Design review of the part built by this model. Coordinates are the model's own, in mm. Face numbers are marked on the shaded views. A direction names the side the tool comes from. Coordinates: 2 decimals unless noted, no trailing zeros. Write each loop counter-clockwise with the first axis right and the second up, starting at its lowest first coordinate (ties: lowest second). Pieces come first, ordered by that corner, then holes.
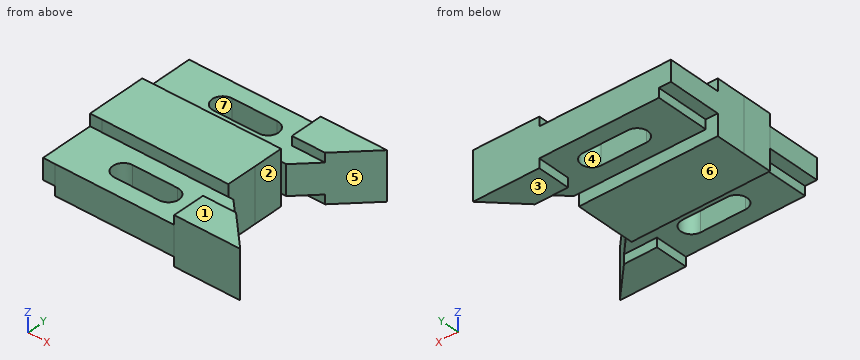
```python
from build123d import *

# Parameters (mm, degrees)
F0_W     = 6.35
F0_H     = 28.575
F1_DEPTH = 28.448
F3_DEPTH = 1.524
F4_DEPTH = 1.524
F5_DEPTH = 6.35
F6_DEPTH = 11.176
F7_DEPTH = 11.176
F2_W     = 6.35
F2_H     = 28.575
F8_DEPTH = 6.35


with BuildPart() as f1:
    # F0 (on Top) → F1 (new body)
    with BuildSketch(Plane.XY):
        Polygon((6.53696, 60.324607), (0.18696, 60.324607), (0.18696, 44.449607), (0.120189, 28.574747), (6.470133, 28.548039), (73.525377, 28.265996), (73.592798, 44.295231), (73.592798, 60.324607), align=None)
        Polygon((69.78296, 88.899607), (6.53696, 88.899607), (6.53696, 60.324607), (73.592798, 60.324607), (76.25996, 60.324607), (87.30896, 71.373607), (69.78296, 71.373607), align=None)
        with BuildLine():
            ThreePointArc((30.41296, 69.024107), (24.82496, 74.612107), (30.41296, 80.200107))
            Line((30.41296, 80.200107), (54.28896, 80.200107))
            ThreePointArc((54.28896, 80.200107), (59.87696, 74.612107), (54.28896, 69.024107))
            Line((54.28896, 69.024107), (30.41296, 69.024107))
        make_face(mode=Mode.SUBTRACT)
        with Locations((3.36196, 74.612107)):
            Rectangle(F0_W, F0_H)
        Polygon((73.525377, 28.265996), (6.470133, 28.548039), (6.349944, -0.026709), (69.595384, -0.292727), (69.6691, 17.233118), (87.194945, 17.159402), (76.192516, 28.254778), align=None)
        with BuildLine():
            Line((54.138112, 8.471865), (30.262323, 8.57229))
            ThreePointArc((30.262323, 8.57229), (24.697876, 14.183744), (30.309331, 19.748191))
            Line((30.309331, 19.748191), (54.185119, 19.647767))
            ThreePointArc((54.185119, 19.647767), (59.749566, 14.036312), (54.138112, 8.471865))
        make_face(mode=Mode.SUBTRACT)
        Polygon((69.6691, 17.233118), (69.595384, -0.292727), (104.647074, -0.440158), (87.194945, 17.159402), align=None)
        Polygon((6.470133, 28.548039), (0.120189, 28.574747), (0, 0), (6.349944, -0.026709), align=None)
        Polygon((104.83496, 88.899607), (69.78296, 88.899607), (69.78296, 71.373607), (87.30896, 71.373607), align=None)
    extrude(amount=F1_DEPTH)

    # F2 (on face) → F3 (cut)
    with BuildSketch(Plane.XY.offset(28.448)):
        Polygon((104.647074, -0.440158), (87.194945, 17.159402), (69.6691, 17.233118), (69.595384, -0.292727), align=None)
        Polygon((69.78296, 71.373607), (87.30896, 71.373607), (104.83496, 88.899607), (69.78296, 88.899607), align=None)
    extrude(amount=-F3_DEPTH, mode=Mode.SUBTRACT)

    # F0 (on Top) → F4 (cut)
    with BuildSketch(Plane.XY):
        Polygon((69.6691, 17.233118), (69.595384, -0.292727), (104.647074, -0.440158), (87.194945, 17.159402), align=None)
        Polygon((104.83496, 88.899607), (69.78296, 88.899607), (69.78296, 71.373607), (87.30896, 71.373607), align=None)
    extrude(amount=F4_DEPTH, mode=Mode.SUBTRACT)

    # F0 (on Top) → F5 (cut)
    with BuildSketch(Plane.XY):
        Polygon((73.525377, 28.265996), (6.470133, 28.548039), (6.349944, -0.026709), (69.595384, -0.292727), (69.6691, 17.233118), (87.194945, 17.159402), (76.192516, 28.254778), align=None)
        with BuildLine():
            Line((54.138112, 8.471865), (30.262323, 8.57229))
            ThreePointArc((30.262323, 8.57229), (24.697876, 14.183744), (30.309331, 19.748191))
            Line((30.309331, 19.748191), (54.185119, 19.647767))
            ThreePointArc((54.185119, 19.647767), (59.749566, 14.036312), (54.138112, 8.471865))
        make_face(mode=Mode.SUBTRACT)
        Polygon((69.78296, 88.899607), (6.53696, 88.899607), (6.53696, 60.324607), (73.592798, 60.324607), (76.25996, 60.324607), (87.30896, 71.373607), (69.78296, 71.373607), align=None)
        with BuildLine():
            ThreePointArc((30.41296, 69.024107), (24.82496, 74.612107), (30.41296, 80.200107))
            Line((30.41296, 80.200107), (54.28896, 80.200107))
            ThreePointArc((54.28896, 80.200107), (59.87696, 74.612107), (54.28896, 69.024107))
            Line((54.28896, 69.024107), (30.41296, 69.024107))
        make_face(mode=Mode.SUBTRACT)
        Polygon((6.470133, 28.548039), (0.120189, 28.574747), (0, 0), (6.349944, -0.026709), align=None)
        with Locations((3.36196, 74.612107)):
            Rectangle(F0_W, F0_H)
    extrude(amount=F5_DEPTH, mode=Mode.SUBTRACT)

    # F0 (on Top) → F6 (join)
    with BuildSketch(Plane.XY):
        Polygon((6.470133, 28.548039), (0.120189, 28.574747), (0, 0), (6.349944, -0.026709), align=None)
        with Locations((3.36196, 74.612107)):
            Rectangle(F0_W, F0_H)
    extrude(amount=F6_DEPTH)

    # F0 (on Top) → F7 (cut)
    with BuildSketch(Plane.XY):
        Polygon((6.470133, 28.548039), (0.120189, 28.574747), (0, 0), (6.349944, -0.026709), align=None)
        with Locations((3.36196, 74.612107)):
            Rectangle(F0_W, F0_H)
    extrude(amount=F7_DEPTH, mode=Mode.SUBTRACT)

    # F2 (on face) → F8 (cut)
    with BuildSketch(Plane.XY.offset(28.448)):
        Polygon((69.6691, 17.233118), (87.194945, 17.159402), (76.192516, 28.254778), (73.525377, 28.265996), (6.470133, 28.548039), (6.349944, -0.026709), (69.595384, -0.292727), align=None)
        with BuildLine():
            Line((30.309331, 19.748191), (54.185119, 19.647767))
            ThreePointArc((54.185119, 19.647767), (59.749566, 14.036312), (54.138112, 8.471865))
            Line((54.138112, 8.471865), (30.262323, 8.57229))
            ThreePointArc((30.262323, 8.57229), (24.697876, 14.183744), (30.309331, 19.748191))
        make_face(mode=Mode.SUBTRACT)
        Polygon((6.53696, 60.324607), (73.592798, 60.324607), (76.25996, 60.324607), (87.30896, 71.373607), (69.78296, 71.373607), (69.78296, 88.899607), (6.53696, 88.899607), align=None)
        with BuildLine():
            ThreePointArc((30.41296, 69.024107), (24.82496, 74.612107), (30.41296, 80.200107))
            Line((30.41296, 80.200107), (54.28896, 80.200107))
            ThreePointArc((54.28896, 80.200107), (59.87696, 74.612107), (54.28896, 69.024107))
            Line((54.28896, 69.024107), (30.41296, 69.024107))
        make_face(mode=Mode.SUBTRACT)
        Polygon((0, 0), (6.349944, -0.026709), (6.470133, 28.548039), (0.120189, 28.574747), align=None)
        with Locations((3.36196, 74.612107)):
            Rectangle(F2_W, F2_H)
    extrude(amount=-F8_DEPTH, mode=Mode.SUBTRACT)


solid = f1.part
```
(1) Consider section A-A (z = 3.5). Give the boundary of the cut face in (x, y).
(2) Consider section C-C (z = 14). Give the boundary of the cut face in (x, y).
(3) Wall thickness on line 1 (Y direction, x = 74.5, z = 11.75); line 2 (Y direction, x = 49, z = 17.5); line 3 (Z direction, x = 96.5, y = 85.5): over which ranges is each line inside the solid? List them lowest first.
(4) Mouldability with a two-part tool opening along X and no side actions: class the marked faces 5, 6 and 7 as +X half, -X half, draft (parallel to the pull), parting line (faces both ways), or undercut.
(5) Insertion check: pin 1 Ø3 at (y, z) = (65.5, 19.5) entering from -X; pin 2 Ø2.5 at (y, z) = (78.5, 4.5) entering from -X; pin 3 Ø10 at (x, y) = (81.5, 55) entering from -Z; pin 4 Ø9 at (x, y) = (81, 76.5) entering from +Z. Each pin has a flat end and moves straight along its axis. Give the tip position at first contact, or say it passes through.
(6) Consider section D-D (y = 74.5). Give the boundary of the cut face in (x, z), plus the area to 3 significant figures.
(7) Consider section B-B (x = 37). Give the boundary of the cut face in (y, z), plus the area to 3 significant figures.
(8) For the marked faces 1, 2, 3 and 4, list the 3-axis set-ups (+Z, -Z, +X, -X, +Y, -Y) from which the entire face can be reached by the end or side of a thin tool; tool diameter is ignored.
Results:
1. outline: (0.12, 28.57) - (6.47, 28.55) - (73.53, 28.27) - (73.59, 44.3) - (73.59, 60.32) - (0.19, 60.32) - (0.19, 44.45) - close; (69.6, -0.29) - (104.65, -0.44) - (87.19, 17.16) - (69.67, 17.23) - close; (69.78, 71.37) - (87.31, 71.37) - (104.83, 88.9) - (69.78, 88.9) - close
2. outline: (0, 0) - (104.65, -0.44) - (76.19, 28.25) - (73.53, 28.27) - (73.59, 44.3) - (73.59, 60.32) - (76.26, 60.32) - (104.83, 88.9) - (0.19, 88.9) - (0.19, 44.45) - close; hole (30.26, 8.57) - (54.14, 8.47) arc R5.59 ccw to (54.19, 19.65) - (30.31, 19.75) arc R5.59 ccw to start; hole (30.41, 69.02) - (54.29, 69.02) arc R5.59 ccw to (54.29, 80.2) - (30.41, 80.2) arc R5.59 ccw to start
3. line 1: y = -0.31 to 28.26, 60.32 to 88.9
3. line 2: y = -0.21 to 8.49, 19.67 to 69.02, 80.2 to 88.9
3. line 3: z = 1.52 to 26.92
4. face 5: +X half
4. face 6: draft
4. face 7: undercut
5. pin 1: stops at x = 0.19
5. pin 2: stops at x = 69.78
5. pin 3: passes through
5. pin 4: stops at z = 26.92
6. outline: (0.19, 11.18) - (6.54, 11.18) - (6.54, 6.35) - (24.83, 6.35) - (24.83, 22.1) - (0.19, 22.1) - close; (59.88, 6.35) - (69.78, 6.35) - (69.78, 1.52) - (90.44, 1.52) - (90.44, 26.92) - (69.78, 26.92) - (69.78, 22.1) - (59.88, 22.1) - close
6. area: 1,040 mm2
7. outline: (-0.16, 6.35) - (8.54, 6.35) - (8.54, 22.1) - (-0.16, 22.1) - close; (19.72, 6.35) - (28.42, 6.35) - (28.42, 0) - (60.32, 0) - (60.32, 6.35) - (69.02, 6.35) - (69.02, 22.1) - (60.32, 22.1) - (60.32, 28.45) - (28.42, 28.45) - (28.42, 22.1) - (19.72, 22.1) - close; (80.2, 6.35) - (88.9, 6.35) - (88.9, 22.1) - (80.2, 22.1) - close
7. area: 1,460 mm2
8. face 1: +Z, +X, -X, -Y
8. face 2: +Z, -Z, +X
8. face 3: -Z, +X, -X, +Y
8. face 4: +Z, -Z
